The model under review builds one solid part; all positions refer to its coordinate system, in mm. Face numbers are marked on the shaded views. Round coordinates to 2 decimals unless told otherwise and drop trailing zeros. Order: outer loops, then holes, each group sorted by start corner. A loop starts at its lowest first (then second) coordinate and runs counter-clockwise, first axis right, second up. Notation, with made-up numbers: M 17,-29 L 24,-29 A32 ccw 24,3 Z; hole C -11.5,-15 d3. An arc over 180 degrees is marked long. Answer as a JSON object with one key per item and string values. Group by question number.
1) Consider section B-B, the plane y = 34.5. Write out the cut boundary in (x, z), then the cut area to 3 significant figures.
2) To check wall thickness, follow line 1 (Z direction, x = 0, y = 21.5); line 2 (Y direction, x = -3.75, z = 4.25); line 3 (Z direction, x = 2.75, y = 34). State the ranges of each line that lie inside material, in increasing order.
3) Consider section A-A, the plane x = 1.25. Write out the cut boundary in (y, z).
4) Insertion check: pin 1 Ø3.5 at (x, z) = (-2.5, 1) entering from -Y; pin 2 Ø4 at (x, y) = (-4.5, 44) entering from -Z; pin 3 Ø2 at (x, z) = (3.5, 3.5) entering from -Y. Each pin has a flat end and moves straight along its axis. Give the tip position at first contact, or say it passes through.
5) The part is to be moulded in two halves that separate along X. For the marked faces 1, 2, 3 and 4, say which applies: +X half, -X half, draft (parallel to the pull), parting line (faces both ways), or undercut.
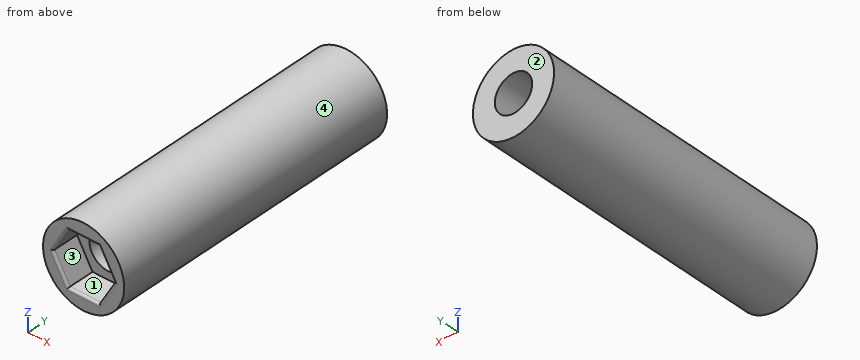
Autodesk Inventor part; units mm, degrees
ref_plane "YZ Plane" through (0, 0, 0) normal (1, 0, 0) x (0, 1, 0)
ref_plane "XZ Plane" through (0, 0, 0) normal (0, 1, 0) x (-1, 0, 0)
ref_plane "XY Plane" through (0, 0, 0) normal (0, 0, 1) x (1, 0, 0)
sketch "Sketch1" plane through (0, 0, 0) normal (0, 1, 0) x (-1, 0, 0)
  circle A0 centre (0, 0) radius 3.91
  circle A1 centre (0, 0) radius 8.5
  line L0 (5.7735, 0) -> (2.8868, -5) construction
  line L1 (2.8868, -5) -> (-2.8868, -5) construction
  line L2 (-2.8868, -5) -> (-5.7735, 0) construction
  line L3 (-5.7735, 0) -> (-2.8868, 5) construction
  line L4 (-2.8868, 5) -> (2.8868, 5) construction
  line L5 (2.8868, 5) -> (5.7735, 0) construction
  line L6 (3.2332, -5.6) -> (6.4663, 0)
  line L7 (6.4663, 0) -> (3.2332, 5.6)
  line L8 (3.2332, 5.6) -> (-3.2332, 5.6)
  line L9 (-3.2332, 5.6) -> (-6.4663, 0)
  line L10 (-6.4663, 0) -> (-3.2332, -5.6)
  line L11 (-3.2332, -5.6) -> (3.2332, -5.6)
  dimension "d0" = 7.82
  dimension "d4" = 10
  dimension "d5" = 0.6
  dimension "d6" = 17
extrude "Extrusion1" add sketch "Sketch1" along normal blind 62.6 contours A1 | L11 L10 L9 L8 L7 L6
extrude "Extrusion2" cut sketch "Sketch1" along normal blind 5.8 contours L11 L10 L9 L8 L7 L6
fillet "Fillet1" radius 0.5 6 edges at (-4.8497, 0, -2.8) (0, 0, -5.6) (4.8497, 0, -2.8) (4.8497, 0, 2.8) (0, 0, 5.6) (-4.8497, 0, 2.8)
properties part number "GenevaPin" material "ABS Plastic"
Results list:
{
 "1": {"outline": "C 0,0 d17; hole C 0,0 d7.82", "area": "179 mm^2"},
 "2": {"line 1": "-8.5 to -3.91, 3.91 to 8.5", "line 2": "5.8 to 62.6", "line 3": "-8.04 to -2.78, 2.78 to 8.04"},
 "3": {"outline": "M 0,-8.41 L 62.6,-8.41 L 62.6,-3.7 L 5.8,-3.7 L 5.8,-5.6 L 0.5,-5.6 A0.5 ccw 0,-6.1 Z; M 0,6.1 A0.5 ccw 0.5,5.6 L 5.8,5.6 L 5.8,3.7 L 62.6,3.7 L 62.6,8.41 L 0,8.41 Z"},
 "4": {"pin 1": "y = 5.8", "pin 2": "z = -8.12", "pin 3": "y = 0.11"},
 "5": {"face 1": "undercut", "face 2": "draft", "face 3": "undercut", "face 4": "parting line"}
}
